```python
from build123d import *

# Parameters (mm, degrees)
F0_W     = 105
F0_H     = 305
F1_DEPTH = 100
F2_T     = -2.5


with BuildPart() as f1:
    # F0 (on Top) → F1 (new body)
    with BuildSketch(Plane.XY):
        Rectangle(F0_W, F0_H)
    extrude(amount=F1_DEPTH)

    # F2
    f2_openings = [f1.faces().sort_by_distance(p)[0] for p in [
        (0, 0, 100),
        (52.5, 0, 50),
        (0, -152.5, 50),
    ]]
    offset(amount=F2_T, openings=f2_openings)


solid = f1.part
```
Geometry: final body of the model. Coordinates: model frame, mm. A direction names the side the tool comes from. Round coordinates to 2 decimals unless told otherwise and drop trailing zeros. Loops run counter-clockwise (first coordinate to the right, second up) from the corner with the lowest first, then second, coordinate; pieces in that order, holes last. Notation, with made-up numbers: (89.25, -7.75) -> (132.25, -7.75) arc R19 cw to (132.25, 6.25) -> close; hole circle Ø7 at (84.25, 89.5). An arc over 180 degrees is marked (long way). Use one line per item in the form item = value. Start each with the question number.
1) Section B-B on x = 36. Output: boundary loops of the cut face in (y, z).
2) Line query: L1, parallel to X at y = -3.5, z = 43; L2, parallel to Y at x = -47, z = 13; L3, parallel to Z at x = 39, y = 95. Output: solid intervals per line, ascending.
3) Section A-A on z = 67. Output: boundary loops of the cut face in (x, y).
4) First-contact query: P1, Ø1, axis at y = 119.5, z = 23, coming from the +X side; P2, Ø12, axis at x = -21.5, z = 29, coming from the -Y side. Flat tips, straight axial feed; report the tip coordinate or a pass-through.
5) Access query for faces 1 (the flat face through (1, 150, 51)), 2 (the flat face through (-1, 152.5, 49)). Directions: +Z, -Z, +X, -X, +Y, -Y. A direction counts if a zero-diameter tool reaches every point of the face in a straight line with its end or side. Return the directions, or none.
Response:
q1.outline = (-152.5, 0) -> (152.5, 0) -> (152.5, 100) -> (150, 100) -> (150, 2.5) -> (-152.5, 2.5) -> close
q2.L1 = -52.5 to -50
q2.L2 = 150 to 152.5
q2.L3 = 0 to 2.5
q3.outline = (-52.5, -152.5) -> (-50, -152.5) -> (-50, 150) -> (52.5, 150) -> (52.5, 152.5) -> (-52.5, 152.5) -> close
q4.P1 = -50
q4.P2 = 150
q5.face_1 = +Z, +X, -Y
q5.face_2 = +Z, -Z, +X, -X, +Y
